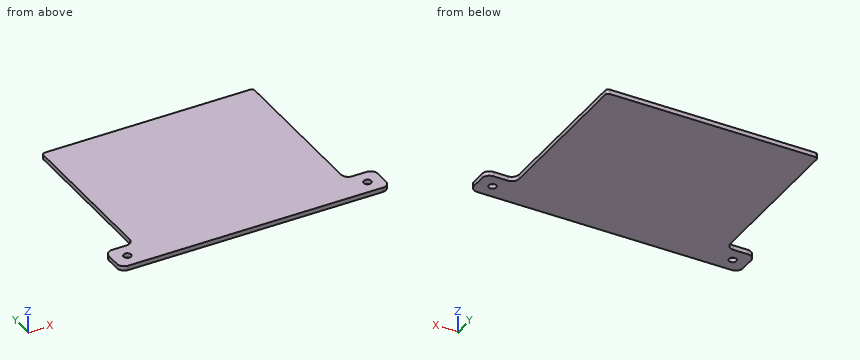
from build123d import *

# Parameters (mm, degrees)
SKETCH1_W           = 20
SKETCH1_H           = 20
SKETCH1_R           = 2.6
SKETCH1_W_2         = 146.5
SKETCH1_H_2         = 133.75
BOSS_EXTRUDE1_DEPTH = 3.175
FILLET2_R           = 5
FILLET3_R           = 2


with BuildPart() as part:
    # Sketch1 → Boss-Extrude1 (new body)
    with BuildSketch(Plane.XY):
        with Locations((-83.25, -56.875)):
            Rectangle(SKETCH1_W, SKETCH1_H)
        with Locations((-83.25, -56.875)):
            Circle(SKETCH1_R, mode=Mode.SUBTRACT)
        Rectangle(SKETCH1_W_2, SKETCH1_H_2)
        with Locations((83.25, -56.875)):
            Rectangle(SKETCH1_W, SKETCH1_H)
        with Locations((83.25, -56.875)):
            Circle(SKETCH1_R, mode=Mode.SUBTRACT)
    extrude(amount=BOSS_EXTRUDE1_DEPTH)

    # Fillet2
    fillet2_edges = [part.edges().sort_by_distance(p)[0] for p in [
        (-73.25, -46.875, 1.5875),
        (73.25, -46.875, 1.5875),
        (93.25, -46.875, 1.5875),
        (93.25, -66.875, 1.5875),
        (-93.25, -66.875, 1.5875),
        (-93.25, -46.875, 1.5875),
    ]]
    fillet(fillet2_edges, radius=FILLET2_R)

    # Fillet3
    fillet3_edges = [part.edges().sort_by_distance(p)[0] for p in [
        (-73.25, 66.875, 1.5875),
        (73.25, 66.875, 1.5875),
    ]]
    fillet(fillet3_edges, radius=FILLET3_R)


solid = part.part
Can you work these out from the model? Positions are in its coordinate system, mm. Give positions to 0.01 mm unless a question says otherwise; leave off trailing zeros. Order: outer loops, then holes, each group sorted by start corner. A loop starts at its lowest first (then second) coordinate and runs counter-clockwise, first axis right, second up. Notation, with made-up numbers: M -27.75,34.5 L -16.75,34.5 A7 ccw -16.75,44.5 Z; hole C 53,61 d3. An arc over 180 degrees is marked long. Use one line per item in the form item = value. Start each with the question number.
Item 1: If we section it at B-B (z = 2.45): Write out the boundary of the cut face in (x, y) (3 decimals), then the cut area to 3 significant figures.
Item 2: If we section it at A-A (x = 83.25): Write out the boundary of the cut face in (y, z) (3 decimals).
Item 3: If we section it at C-C (y = 36.5): Write out the boundary of the cut face in (x, z) (3 decimals).
Item 4: Will these pins go through, and if not, where does the flat tip stop? pin 1 Ø1 at (y, z) = (-3, 1) entering from -X; pin 2 Ø1.6 at (x, z) = (-84.5, 1.5) entering from +Y (3 decimals).
Item 5: If I drill on line 1 along X through (y, z) = (-57, 1.1); line 2 along Y through (x, z) = (-83.25, 1.65) (3 decimals); line 3 along X through (y, z) = (12, 1.9), over which ranges is the centre line in solid material (lowest first)?
Outcome:
q1.outline = M -93.25,-61.875 A5 ccw -88.25,-66.875 L 88.25,-66.875 A5 ccw 93.25,-61.875 L 93.25,-51.875 A5 ccw 88.25,-46.875 L 78.25,-46.875 A5 cw 73.25,-41.875 L 73.25,64.875 A2 ccw 71.25,66.875 L -71.25,66.875 A2 ccw -73.25,64.875 L -73.25,-41.875 A5 cw -78.25,-46.875 L -88.25,-46.875 A5 ccw -93.25,-51.875 Z; hole C -83.25,-56.875 d5.2; hole C 83.25,-56.875 d5.2
q1.area = 20,300 mm2
q2.outline = M -66.875,0 L -59.475,0 L -59.475,3.175 L -66.875,3.175 Z; M -54.275,0 L -46.875,0 L -46.875,3.175 L -54.275,3.175 Z
q3.outline = M -73.25,0 L 73.25,0 L 73.25,3.175 L -73.25,3.175 Z
q4.pin_1 = -73.25
q4.pin_2 = -46.875
q5.line_1 = -93.25 to -85.85, -80.65 to 80.65, 85.85 to 93.25
q5.line_2 = -66.875 to -59.475, -54.275 to -46.875
q5.line_3 = -73.25 to 73.25
